Can you work these out from the model? Positions are in its coordinate system, mm. Round coordinates to 2 decimals unless told otherwise and drop trailing zeros. Loops run counter-clockwise (first coordinate to the right, second up) from the corner with the lowest first, then second, coordinate; pieces in that order, holes last. Notation, with made-up numbers: (5, 78.25) -> (56, 78.25) arc R13 ccw to (56, 83.25) -> close; hole circle Ø2 at (41, -27). An arc over 180 degrees is marked (long way). Write each question's results on one line, items separated by ' | '.
Autodesk Inventor part; units mm, degrees
ref_plane "YZ Plane" through (0, 0, 0) normal (1, 0, 0) x (0, 1, 0)
ref_plane "XZ Plane" through (0, 0, 0) normal (0, 1, 0) x (-1, 0, 0)
ref_plane "XY Plane" through (0, 0, 0) normal (0, 0, 1) x (1, 0, 0)
sketch "Sketch1" plane through (0, 0, 0) normal (0, 0, 1) x (1, 0, 0)
  arc A0 (103.6702, 18.7694) -> (117.1276, 18.7694) centre (110.3989, 29.5404) ccw
  line L0 (103.6702, 40.3608) -> (103.6702, 29.5898)
  line L1 (117.1276, 40.3608) -> (117.1276, 29.5898)
  line L2 (95.2163, 29.5898) -> (125.5815, 29.5898)
  arc A1 (117.1276, 40.3608) -> (103.6702, 40.3608) centre (110.3989, 29.5898) ccw
  point P0 (0, 0)
  point P1 (110.3989, 16.8404)
  dimension "d44" = 21.6408
  dimension "d45" = 12.7
  dimension "d46" = 12.7
revolve "Revolution1" add sketch "Sketch1" angle 360 about axis through (95.2163, 29.5898, 0) along (1, 0, 0)
sketch "Sketch2" plane through (117.1276, 29.5898, 0) normal (1, 0, 0) x (0, 0, -1)
  circle A0 centre (0, 0) radius 10.771
  point P0 (0, -29.5898)
hole "Hole1" at (117.1276, 29.5898, 0) direction (-1, 0, 0) diameter 9.5377 depth 25.4 tip angle 118
chamfer "Chamfer1" distance 0.254 angle 45 1 edges at (117.1276, 29.5898, 4.7689)
equation "\"d45\" = d46"
properties part number "FM1406P"
1. Will these pins go through, and if not, where does the flat tip stop? pin 1 (1.5 mm diameter, centred on x = 111.5, y = 21.5, fed in from -Z); pin 2 (8 mm diameter, centred on x = 108.5, y = 25, fed in from +Z); pin 3 (5 mm diameter, centred on x = 112.5, y = 25.5, fed in from -Z).
Final values:
pin 1: z = -10.31 | pin 2: z = 12.66 | pin 3: z = -12.53
2. If we section it at B-B (x = 107.25): List the corners of the cut face in (y, z) for me.
Final values:
outline: circle Ø24.61 at (29.59, 0); hole circle Ø9.54 at (29.59, 0)
3. We'd pull the mould along Y, two halves only. Please class faces 1 (the face through (110.18, 33.82, -2.2)), 2 (the face through (103.67, 34.2, -2.2)): pulls with the +Y half, pulls with the -Y half, needs draft (parallel to the pull), parting line crosses it, or undercut.
Final values:
face 1: undercut | face 2: needs draft
4. Please list where these lines run through material, in increasing order: line 1 (Z direction, x = 115.5, y = 29); line 2 (Z direction, x = 112, y = 30.5); line 3 (Y direction, x = 106.5, z = 0). Write a range as from..to.
Final values:
line 1: -11.62..-4.73, 4.73..11.62 | line 2: -12.57..-4.68, 4.68..12.57 | line 3: 17.5..24.82, 34.36..41.68
5. If we section it at D-D (z = 7.25): List the corners of the cut face in (x, y) for me, then the cut area to 3 significant figures.
Final values:
outline: (103.67, 21.62) arc R10.43 ccw to (117.13, 21.62) -> (117.13, 37.56) arc R10.43 ccw to (103.67, 37.56) -> close | area: 260 mm2
6. If we section it at C-C (y = 37.25): List the corners of the cut face in (x, z) for me, then the cut area to 3 significant figures.
Final values:
outline: (103.67, -7.57) arc R10.13 ccw to (117.13, -7.57) -> (117.13, 7.57) arc R10.13 ccw to (103.67, 7.57) -> close | area: 251 mm2
7. If we section it at A-A (z = 0): List the corners of the cut face in (x, y) for me.
Final values:
outline: (103.67, 18.82) arc R12.7 ccw to (117.13, 18.82) -> (117.13, 24.57) -> (116.87, 24.82) -> (103.67, 24.82) -> close; (103.67, 34.36) -> (116.87, 34.36) -> (117.13, 34.61) -> (117.13, 40.36) arc R12.7 ccw to (103.67, 40.36) -> close
